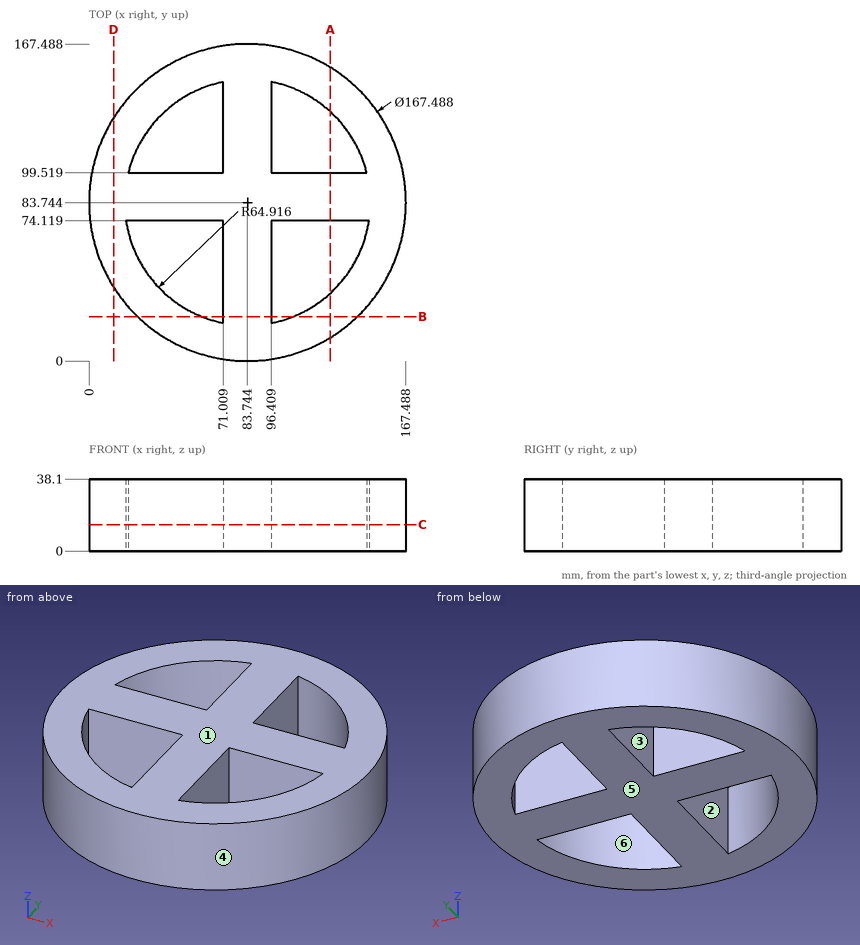
Answer from the drawing. Dimensions are ordinates in mm from the lowest x, y and z of the part. A direction names the side the tool comes from. Give positions to 0.01 mm unless a question says otherwise; leave off trailing zeros. Order: outer loops, then holes, each group sorted by start corner. A loop starts at its lowest first (then second) coordinate and runs counter-clockwise, first axis right, second up.
(1) Find section A-A (x = 127.5). Give the vertices of the cut face in (y, z).
(2) Straight lines are drawn through the part: L1, parallel to Y at x = 115.5, z = 13.5 (1 decimal); L2, parallel to X at y = 57.5, z = 36; L3, parallel to Y at x = 132.5, z = 25.5 (1 decimal). For each, find the intervals that lie inside material, in ascending order.
(3) For a pull along Y with two mould halves and no side action, classify the marked faces 3, 4, 5 and 6 as released by +Y, released by -Y, zero draft, split by the parting line, or undercut.
(4) Find section D-D (x = 13). Give the vertices of the cut face in (y, z), plus the area to 4 significant figures.
(5) Find section B-B (y = 23.5). Give the vertices of the cut face in (x, z) (1 decimal).
(6) Given pin 1 (4 mm diameter, centred on x = 108, z = 28, fed in from -Y); pin 2 (11.5 mm diameter, centred on x = 47, z = 23.5, fed in from -Y); pin 3 (19 mm diameter, centred on x = 128.5, z = 27.5, fed in from -Y), each flat-ended and moving along its own axis, determine where each tip first touches the part or whether it passes through.
(7) Find section C-C (z = 14). Give the vertices of the cut face in (x, y) (1 decimal).
(8) For the marked faces 1 and 2, determine the directions among +Z, -Z, +X, -X, +Y, -Y from which every point of the face is accessible in a straight line to the end or side of a thin tool.
Result sheet:
1. outline: (12.34, 0) - (35.79, 0) - (35.79, 38.1) - (12.34, 38.1) - close; (74.12, 0) - (99.52, 0) - (99.52, 38.1) - (74.12, 38.1) - close; (131.7, 0) - (155.15, 0) - (155.15, 38.1) - (131.7, 38.1) - close
2. L1: y = 6.3 to 27.1, 74.1 to 99.5, 140.4 to 161.2
2. L2: x = 4.22 to 24.37, 71.01 to 96.41, 143.12 to 163.27
2. L3: y = 15.7 to 40.9, 74.1 to 99.5, 126.6 to 151.8
3. face 3: undercut
3. face 4: split by the parting line
3. face 5: zero draft
3. face 6: undercut
4. outline: (38.93, 0) - (128.56, 0) - (128.56, 38.1) - (38.93, 38.1) - close
4. area: 3,415 mm2
5. outline: (25.6, 0) - (59.6, 0) - (59.6, 38.1) - (25.6, 38.1) - close; (71, 0) - (96.4, 0) - (96.4, 38.1) - (71, 38.1) - close; (107.9, 0) - (141.9, 0) - (141.9, 38.1) - (107.9, 38.1) - close
6. pin 1: stops at y = 3.01
6. pin 2: stops at y = 5.95
6. pin 3: stops at y = 7.78
7. outline: circle Ø167.5 at (83.7, 83.7); hole (19.5, 74.1) arc R64.9 ccw to (71, 20.1) - (71, 74.1) - close; hole (20.8, 99.5) - (71, 99.5) - (71, 147.4) arc R64.9 ccw to start; hole (96.4, 20.1) arc R64.9 ccw to (147.9, 74.1) - (96.4, 74.1) - close; hole (96.4, 99.5) - (146.7, 99.5) arc R64.9 ccw to (96.4, 147.4) - close
8. face 1: +Z, +X, -X, +Y, -Y
8. face 2: +Z, -Z
